CAD build for the part. Positions are in the model's coordinates, mm. Face numbers are marked on the shaded views. Give positions to 0.01 mm unless a question says otherwise; leave off trailing zeros. Write each loop counter-clockwise with the first axis right and the second up, starting at its lowest first coordinate (ties: lowest second). Pieces come first, ordered by that corner, then holes. Notation, with made-up numbers: (-20.5, 23) -> (5.5, 23) arc R30 ccw to (5.5, 58) -> close; hole circle Ø4 at (9, 15.25). An arc over 180 degrees is marked (long way). Use one line per item in the form item = value. Start each with the question number.
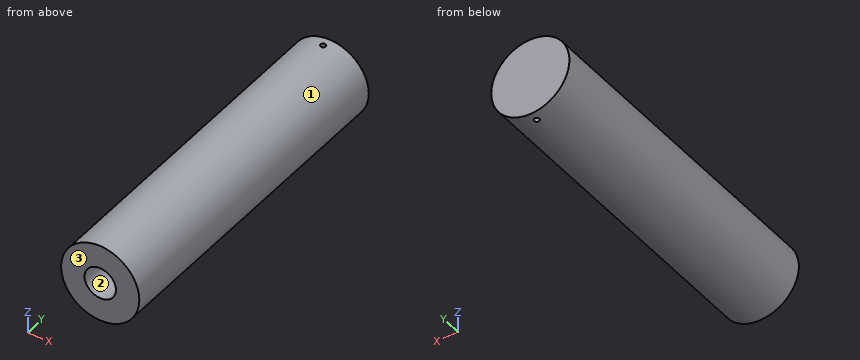
from build123d import *

# Parameters (mm, degrees)
SKETCH1_R                   = 6.35
BOSS_EXTRUDE1_DEPTH         = 53.975
F_1_4_20_TAPPED_HOLE1_D     = 5.1054
F_1_4_20_TAPPED_HOLE1_DEPTH = 25.4
F_1_4_20_TAPPED_HOLE1_TIP   = 1.533816902
F_66_0_033_DIAMETER_HOLE1_D = 0.8382


with BuildPart() as part:
    # Sketch1 → Boss-Extrude1 (new body)
    with BuildSketch(Plane(origin=(0, 0, 0), x_dir=(1, 0, 0), z_dir=(0, 1, 0))):
        Circle(SKETCH1_R)
    extrude(amount=BOSS_EXTRUDE1_DEPTH)

    # 1/4-20 Tapped Hole1
    with Locations(Plane(origin=(0, 0, 0), x_dir=(-1, 0, 0), z_dir=(0, -1, 0))):
        with Locations((0, 0)):
            Hole(F_1_4_20_TAPPED_HOLE1_D / 2, depth=F_1_4_20_TAPPED_HOLE1_DEPTH)
            with Locations((0, 0, -(F_1_4_20_TAPPED_HOLE1_DEPTH + F_1_4_20_TAPPED_HOLE1_TIP / 2))):  # 118° drill point
                Cone(0, F_1_4_20_TAPPED_HOLE1_D / 2, F_1_4_20_TAPPED_HOLE1_TIP, mode=Mode.SUBTRACT)

    # #66 (0.033) Diameter Hole1 (through all)
    with Locations(Plane(origin=(-0.006974239, 52.448108519, 6.34999617), x_dir=(0.999999397, 0, 0.001098305), z_dir=(-0.001098305, 0, 0.999999397))):
        with Locations((0, 0)):
            Hole(F_66_0_033_DIAMETER_HOLE1_D / 2)


solid = part.part
1) Two-plate mould, pull along X, no slides. Class the marked faces 1, 2 and 3: released by +X, released by -X, zero draft, split by the parting line, or undercut.
2) Wall check: line 1 along Z through (x, y) = (0, 11.25); line 2 along Y through (x, z) = (0, 4) (3 decimals); line 3 along Z through (x, y) = (3.75, 38.5). Give the ranges that are in metal, low to high. Write a range as from..to.
3) Cut at B-B (y = 45). Give the cut face in (x, z), and give its area (3 significant figures).
4) Pin check, flat tips, straight feed: pin 1 (1.5 mm diameter, centred on x = -0.5, y = 18.5, fed in from +Z); pin 2 (4 mm diameter, centred on y = 32, z = -3.5, fed in from -X); pin 3 (1 mm diameter, centred on y = 15, z = -4, fed in from -X). Stop position of each tip, or through.
5) Cut at A-A (y = 14). Give the cut face in (x, z).
6) Cut at C-C (x = 5.25). Give the cut face in (y, z) (3 decimals), and give its area (3 significant figures).
Final values:
q1.face_1 = split by the parting line
q1.face_2 = undercut
q1.face_3 = zero draft
q2.line_1 = -6.35..-2.55, 2.55..6.35
q2.line_2 = 0..52.029, 52.867..53.975
q2.line_3 = -5.12..5.12
q3.outline = circle Ø12.7 at (0, 0)
q3.area = 127 mm^2
q4.pin_1 = 6.35
q4.pin_2 = -6.17
q4.pin_3 = -5.3
q5.outline = circle Ø12.7 at (0, 0); hole circle Ø5.11 at (0, 0)
q6.outline = (0, -3.572) -> (53.975, -3.572) -> (53.975, 3.572) -> (0, 3.572) -> close
q6.area = 386 mm^2
